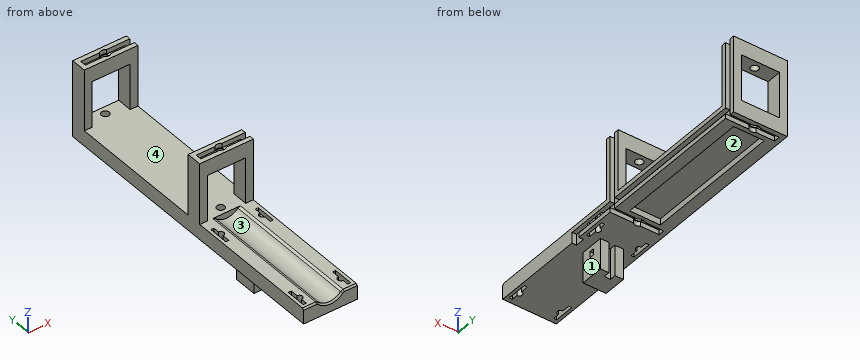
```python
from build123d import *

# Parameters (mm, degrees)
CYLINDER005_R     = 3
CYLINDER005_DEPTH = 3
CYLINDER006_R     = 3
CYLINDER006_DEPTH = 3
CYLINDER002_R     = 2.5
CYLINDER002_DEPTH = 60
BOX010_W          = 30
BOX010_H          = 4
BOX010_DEPTH      = 3
BOX008_W          = 30
BOX008_H          = 4
BOX008_DEPTH      = 3
BOX006_W          = 3
BOX006_H          = 4
BOX006_DEPTH      = 50
BOX004_W          = 3
BOX004_H          = 136
BOX004_DEPTH      = 4
BOX003_W          = 25
BOX003_H          = 220
BOX003_DEPTH      = 30
BOX002_W          = 35
BOX002_H          = 10
BOX002_DEPTH      = 50
BOX021_W          = 3
BOX021_H          = 6
BOX021_DEPTH      = 4
BOX018_W          = 20
BOX018_H          = 90
BOX018_DEPTH      = 4
CYLINDER008_R     = 2
CYLINDER008_DEPTH = 10
CYLINDER009_R     = 2
CYLINDER009_DEPTH = 10
CYLINDER010_R     = 2
CYLINDER010_DEPTH = 10
CYLINDER007_R     = 2
CYLINDER007_DEPTH = 10
BOX015_W          = 2
BOX015_H          = 13
BOX015_DEPTH      = 10
BOX016_W          = 2
BOX016_H          = 13
BOX016_DEPTH      = 10
BOX017_W          = 2
BOX017_H          = 13
BOX017_DEPTH      = 10
BOX014_W          = 2
BOX014_H          = 13
BOX014_DEPTH      = 10
CYLINDER003_R     = 3
CYLINDER003_DEPTH = 3
CYLINDER001_R     = 2.5
CYLINDER001_DEPTH = 60
BOX007_W          = 30
BOX007_H          = 4
BOX007_DEPTH      = 3
BOX005_W          = 3
BOX005_H          = 4
BOX005_DEPTH      = 50
CYLINDER_R        = 10
CYLINDER_DEPTH    = 90
BOX_W             = 35
BOX_H             = 200
BOX_DEPTH         = 10
CHAMFER_SIZE      = 1
BOX023_W          = 4
BOX023_H          = 4
BOX023_DEPTH      = 20
BOX022_W          = 20
BOX022_H          = 3
BOX022_DEPTH      = 4
BOX019_W          = 15
BOX019_H          = 15
BOX019_DEPTH      = 20
CYLINDER004_R     = 3
CYLINDER004_DEPTH = 3
BOX009_W          = 30
BOX009_H          = 4
BOX009_DEPTH      = 3
BOX001_W          = 35
BOX001_H          = 10
BOX001_DEPTH      = 50


with BuildPart() as cilindro005:
    # Cylinder005 → Cylinder005 (new body)
    with BuildSketch(Plane(origin=(17.5, 195, 0), x_dir=(1, 0, 0), z_dir=(0, 0, 1))):
        Circle(CYLINDER005_R)
    extrude(amount=CYLINDER005_DEPTH)


with BuildPart() as cilindro006:
    # Cylinder006 → Cylinder006 (new body)
    with BuildSketch(Plane(origin=(17.5, 195, 47), x_dir=(1, 0, 0), z_dir=(0, 0, 1))):
        Circle(CYLINDER006_R)
    extrude(amount=CYLINDER006_DEPTH)


with BuildPart() as cilindro002:
    # Cylinder002 → Cylinder002 (new body)
    with BuildSketch(Plane(origin=(17.5, 195, -1), x_dir=(1, 0, 0), z_dir=(0, 0, 1))):
        Circle(CYLINDER002_R)
    extrude(amount=CYLINDER002_DEPTH)


with BuildPart() as cubo010:
    # Box010 → Box010 (new body)
    with BuildSketch(Plane(origin=(3, 193, 47), x_dir=(1, 0, 0), z_dir=(0, 0, 1))):
        with Locations((15, 2)):
            Rectangle(BOX010_W, BOX010_H)
    extrude(amount=BOX010_DEPTH)


with BuildPart() as cubo008:
    # Box008 → Box008 (new body)
    with BuildSketch(Plane(origin=(3, 193, 0), x_dir=(1, 0, 0), z_dir=(0, 0, 1))):
        with Locations((15, 2)):
            Rectangle(BOX008_W, BOX008_H)
    extrude(amount=BOX008_DEPTH)


with BuildPart() as cubo006:
    # Box006 → Box006 (new body)
    with BuildSketch(Plane(origin=(32, 193, 0), x_dir=(1, 0, 0), z_dir=(0, 0, 1))):
        with Locations((1.5, 2)):
            Rectangle(BOX006_W, BOX006_H)
    extrude(amount=BOX006_DEPTH)


with BuildPart() as cubo004:
    # Box004 → Box004 (new body)
    with BuildSketch(Plane(origin=(32, 60, 3), x_dir=(1, 0, 0), z_dir=(0, 0, 1))):
        with Locations((1.5, 68)):
            Rectangle(BOX004_W, BOX004_H)
    extrude(amount=BOX004_DEPTH)


with BuildPart() as cubo003:
    # Box003 → Box003 (new body)
    with BuildSketch(Plane(origin=(5, 0, 10), x_dir=(1, 0, 0), z_dir=(0, 0, 1))):
        with Locations((12.5, 110)):
            Rectangle(BOX003_W, BOX003_H)
    extrude(amount=BOX003_DEPTH)


with BuildPart() as cut023:
    # Box002 → Box002 (new body)
    with BuildSketch(Plane(origin=(0, 190, 0), x_dir=(1, 0, 0), z_dir=(0, 0, 1))):
        with Locations((17.5, 5)):
            Rectangle(BOX002_W, BOX002_H)
    extrude(amount=BOX002_DEPTH)

    # Cut002: cut Cubo003
    add(cubo003.part, mode=Mode.SUBTRACT)

    # Cut005: cut Cubo004
    add(cubo004.part, mode=Mode.SUBTRACT)

    # Cut007: cut Cubo006
    add(cubo006.part, mode=Mode.SUBTRACT)

    # Cut011: cut Cubo008
    add(cubo008.part, mode=Mode.SUBTRACT)

    # Cut015: cut Cubo010
    add(cubo010.part, mode=Mode.SUBTRACT)

    # Cut017: cut Cilindro002
    add(cilindro002.part, mode=Mode.SUBTRACT)

    # Cut021: cut Cilindro006
    add(cilindro006.part, mode=Mode.SUBTRACT)

    # Cut023: cut Cilindro005
    add(cilindro005.part, mode=Mode.SUBTRACT)


with BuildPart() as cubo021:
    # Box021 → Box021 (new body)
    with BuildSketch(Plane(origin=(32, 60, 0), x_dir=(1, 0, 0), z_dir=(0, 0, 1))):
        with Locations((1.5, 3)):
            Rectangle(BOX021_W, BOX021_H)
    extrude(amount=BOX021_DEPTH)


with BuildPart() as cubo018:
    # Box018 → Box018 (new body)
    with BuildSketch(Plane(origin=(7.5, 100, 0), x_dir=(1, 0, 0), z_dir=(0, 0, 1))):
        with Locations((10, 45)):
            Rectangle(BOX018_W, BOX018_H)
    extrude(amount=BOX018_DEPTH)


with BuildPart() as cilindro008:
    # Cylinder008 → Cylinder008 (new body)
    with BuildSketch(Plane(origin=(31, 9, 0), x_dir=(1, 0, 0), z_dir=(0, 0, 1))):
        Circle(CYLINDER008_R)
    extrude(amount=CYLINDER008_DEPTH)


with BuildPart() as cilindro009:
    # Cylinder009 → Cylinder009 (new body)
    with BuildSketch(Plane(origin=(31, 77, 0), x_dir=(1, 0, 0), z_dir=(0, 0, 1))):
        Circle(CYLINDER009_R)
    extrude(amount=CYLINDER009_DEPTH)


with BuildPart() as cilindro010:
    # Cylinder010 → Cylinder010 (new body)
    with BuildSketch(Plane(origin=(4, 77, 0), x_dir=(1, 0, 0), z_dir=(0, 0, 1))):
        Circle(CYLINDER010_R)
    extrude(amount=CYLINDER010_DEPTH)


with BuildPart() as cilindro007:
    # Cylinder007 → Cylinder007 (new body)
    with BuildSketch(Plane(origin=(4, 9, 0), x_dir=(1, 0, 0), z_dir=(0, 0, 1))):
        Circle(CYLINDER007_R)
    extrude(amount=CYLINDER007_DEPTH)


with BuildPart() as cubo015:
    # Box015 → Box015 (new body)
    with BuildSketch(Plane(origin=(31, 3, 0), x_dir=(1, 0, 0), z_dir=(0, 0, 1))):
        with Locations((1, 6.5)):
            Rectangle(BOX015_W, BOX015_H)
    extrude(amount=BOX015_DEPTH)


with BuildPart() as cubo016:
    # Box016 → Box016 (new body)
    with BuildSketch(Plane(origin=(2, 70, 0), x_dir=(1, 0, 0), z_dir=(0, 0, 1))):
        with Locations((1, 6.5)):
            Rectangle(BOX016_W, BOX016_H)
    extrude(amount=BOX016_DEPTH)


with BuildPart() as cubo017:
    # Box017 → Box017 (new body)
    with BuildSketch(Plane(origin=(31, 70, 0), x_dir=(1, 0, 0), z_dir=(0, 0, 1))):
        with Locations((1, 6.5)):
            Rectangle(BOX017_W, BOX017_H)
    extrude(amount=BOX017_DEPTH)


with BuildPart() as cubo014:
    # Box014 → Box014 (new body)
    with BuildSketch(Plane(origin=(2, 3, 0), x_dir=(1, 0, 0), z_dir=(0, 0, 1))):
        with Locations((1, 6.5)):
            Rectangle(BOX014_W, BOX014_H)
    extrude(amount=BOX014_DEPTH)


with BuildPart() as cilindro003:
    # Cylinder003 → Cylinder003 (new body)
    with BuildSketch(Plane(origin=(17.5, 95, 0), x_dir=(1, 0, 0), z_dir=(0, 0, 1))):
        Circle(CYLINDER003_R)
    extrude(amount=CYLINDER003_DEPTH)


with BuildPart() as cilindro001:
    # Cylinder001 → Cylinder001 (new body)
    with BuildSketch(Plane(origin=(17.5, 95, -1), x_dir=(1, 0, 0), z_dir=(0, 0, 1))):
        Circle(CYLINDER001_R)
    extrude(amount=CYLINDER001_DEPTH)


with BuildPart() as cubo007:
    # Box007 → Box007 (new body)
    with BuildSketch(Plane(origin=(3, 93, 0), x_dir=(1, 0, 0), z_dir=(0, 0, 1))):
        with Locations((15, 2)):
            Rectangle(BOX007_W, BOX007_H)
    extrude(amount=BOX007_DEPTH)


with BuildPart() as cubo005:
    # Box005 → Box005 (new body)
    with BuildSketch(Plane(origin=(32, 93, 0), x_dir=(1, 0, 0), z_dir=(0, 0, 1))):
        with Locations((1.5, 2)):
            Rectangle(BOX005_W, BOX005_H)
    extrude(amount=BOX005_DEPTH)


with BuildPart() as cilindro:
    # Cylinder → Cylinder (new body)
    with BuildSketch(Plane(origin=(17.5, 0, 16), x_dir=(1, 0, 0), z_dir=(0, 1, 0))):
        Circle(CYLINDER_R)
    extrude(amount=CYLINDER_DEPTH)


with BuildPart() as cut037:
    # Box → Box (new body)
    with BuildSketch(Plane.XY):
        with Locations((17.5, 100)):
            Rectangle(BOX_W, BOX_H)
    extrude(amount=BOX_DEPTH)

    # Cut: cut Cilindro
    add(cilindro.part, mode=Mode.SUBTRACT)

    # Chamfer
    chamfer_edges = [cut037.edges().sort_by_distance(p)[0] for p in [
        (30.25, 0, 10),
        (17.5, 0, 6),
        (4.75, 0, 10),
        (25.5, 45, 10),
        (9.5, 45, 10),
    ]]
    chamfer(chamfer_edges, length=CHAMFER_SIZE)

    # Cut003: cut Cubo004
    add(cubo004.part, mode=Mode.SUBTRACT)

    # Cut008: cut Cubo005
    add(cubo005.part, mode=Mode.SUBTRACT)

    # Cut009: cut Cubo006
    add(cubo006.part, mode=Mode.SUBTRACT)

    # Cut012: cut Cubo007
    add(cubo007.part, mode=Mode.SUBTRACT)

    # Cut013: cut Cubo008
    add(cubo008.part, mode=Mode.SUBTRACT)

    # Cut018: cut Cilindro001
    add(cilindro001.part, mode=Mode.SUBTRACT)

    # Cut019: cut Cilindro002
    add(cilindro002.part, mode=Mode.SUBTRACT)

    # Cut024: cut Cilindro003
    add(cilindro003.part, mode=Mode.SUBTRACT)

    # Cut025: cut Cilindro005
    add(cilindro005.part, mode=Mode.SUBTRACT)

    # Cut028: cut Cubo014
    add(cubo014.part, mode=Mode.SUBTRACT)

    # Cut029: cut Cubo017
    add(cubo017.part, mode=Mode.SUBTRACT)

    # Cut030: cut Cubo016
    add(cubo016.part, mode=Mode.SUBTRACT)

    # Cut031: cut Cubo015
    add(cubo015.part, mode=Mode.SUBTRACT)

    # Cut032: cut Cilindro007
    add(cilindro007.part, mode=Mode.SUBTRACT)

    # Cut033: cut Cilindro010
    add(cilindro010.part, mode=Mode.SUBTRACT)

    # Cut034: cut Cilindro009
    add(cilindro009.part, mode=Mode.SUBTRACT)

    # Cut035: cut Cilindro008
    add(cilindro008.part, mode=Mode.SUBTRACT)

    # Cut036: cut Cubo018
    add(cubo018.part, mode=Mode.SUBTRACT)

    # Cut037: cut Cubo021
    add(cubo021.part, mode=Mode.SUBTRACT)


with BuildPart() as cubo023:
    # Box023 → Box023 (new body)
    with BuildSketch(Plane(origin=(16, 61, -20), x_dir=(1, 0, 0), z_dir=(0, 0, 1))):
        with Locations((2, 2)):
            Rectangle(BOX023_W, BOX023_H)
    extrude(amount=BOX023_DEPTH)


with BuildPart() as cubo022:
    # Box022 → Box022 (new body)
    with BuildSketch(Plane(origin=(8, 56, -7), x_dir=(1, 0, 0), z_dir=(0, 0, 1))):
        with Locations((10, 1.5)):
            Rectangle(BOX022_W, BOX022_H)
    extrude(amount=BOX022_DEPTH)


with BuildPart() as cut039:
    # Box019 → Box019 (new body)
    with BuildSketch(Plane(origin=(10.5, 50, -20), x_dir=(1, 0, 0), z_dir=(0, 0, 1))):
        with Locations((7.5, 7.5)):
            Rectangle(BOX019_W, BOX019_H)
    extrude(amount=BOX019_DEPTH)

    # Cut038: cut Cubo022
    add(cubo022.part, mode=Mode.SUBTRACT)

    # Cut039: cut Cubo023
    add(cubo023.part, mode=Mode.SUBTRACT)


with BuildPart() as cut039_1:
    # Cut039 placement: moved
    add(cut039.part.moved(Location((0, 7, 0))))


with BuildPart() as cilindro004:
    # Cylinder004 → Cylinder004 (new body)
    with BuildSketch(Plane(origin=(17.5, 95, 47), x_dir=(1, 0, 0), z_dir=(0, 0, 1))):
        Circle(CYLINDER004_R)
    extrude(amount=CYLINDER004_DEPTH)


with BuildPart() as cubo009:
    # Box009 → Box009 (new body)
    with BuildSketch(Plane(origin=(3, 93, 47), x_dir=(1, 0, 0), z_dir=(0, 0, 1))):
        with Locations((15, 2)):
            Rectangle(BOX009_W, BOX009_H)
    extrude(amount=BOX009_DEPTH)


with BuildPart() as fusion:
    # Box001 → Box001 (new body)
    with BuildSketch(Plane(origin=(0, 90, 0), x_dir=(1, 0, 0), z_dir=(0, 0, 1))):
        with Locations((17.5, 5)):
            Rectangle(BOX001_W, BOX001_H)
    extrude(amount=BOX001_DEPTH)

    # Cut001: cut Cubo003
    add(cubo003.part, mode=Mode.SUBTRACT)

    # Cut004: cut Cubo004
    add(cubo004.part, mode=Mode.SUBTRACT)

    # Cut006: cut Cubo005
    add(cubo005.part, mode=Mode.SUBTRACT)

    # Cut010: cut Cubo007
    add(cubo007.part, mode=Mode.SUBTRACT)

    # Cut014: cut Cubo009
    add(cubo009.part, mode=Mode.SUBTRACT)

    # Cut016: cut Cilindro001
    add(cilindro001.part, mode=Mode.SUBTRACT)

    # Cut020: cut Cilindro004
    add(cilindro004.part, mode=Mode.SUBTRACT)

    # Cut022: cut Cilindro003
    add(cilindro003.part, mode=Mode.SUBTRACT)

    # Fusion: union Cut023, Cut037, Cut039
    add(cut023.part)
    add(cut037.part)
    add(cut039_1.part)


solid = fusion.part
```
The listing builds one solid part. Answer for the finished solid, in the listing's coordinates (mm). Face numbers are marked on the shaded views. A direction names the side the tool comes from. Give positions to 0.01 mm unless a question says otherwise; leave off trailing zeros. Order: outer loops, then holes, each group sorted by start corner. A loop starts at its lowest first (then second) coordinate and runs counter-clockwise, first axis right, second up. Notation, with made-up numbers: (29, 49.5) -> (33, 49.5) arc R11 cw to (33, 69.5) -> close; hole circle Ø1 at (63, 70). An arc over 180 degrees is marked (long way). Write each question's results on one line, items separated by ' | '.
Q1. The part is cut by section B-B, the plane z = 17.5. Give the vertices of the cut face in (x, y).
Checked values:
outline: (0, 90) -> (5, 90) -> (5, 100) -> (0, 100) -> close; (0, 190) -> (5, 190) -> (5, 200) -> (0, 200) -> close; (30, 90) -> (35, 90) -> (35, 93) -> (32, 93) -> (32, 97) -> (35, 97) -> (35, 100) -> (30, 100) -> close; (30, 190) -> (35, 190) -> (35, 193) -> (32, 193) -> (32, 197) -> (35, 197) -> (35, 200) -> (30, 200) -> close
Q2. Determine the mould class of the marked faces 1 and 2 for opening direction X: pulls with the +X half, pulls with the -X half, needs draft (parallel to the pull), parting line crosses it, or undercut.
Checked values:
face 1: pulls with the +X half | face 2: undercut
Q3. The part is cut by section C-C, the plane y = 195. Give the vertices of the cut face in (x, z), and give its area (3 significant figures).
Checked values:
outline: (0, 0) -> (3, 0) -> (3, 3) -> (15, 3) -> (15, 10) -> (5, 10) -> (5, 40) -> (15, 40) -> (15, 47) -> (3, 47) -> (3, 50) -> (0, 50) -> close; (20, 3) -> (32, 3) -> (32, 47) -> (20, 47) -> (20, 40) -> (30, 40) -> (30, 10) -> (20, 10) -> close | area: 606 mm^2
Q4. The part is cut by section D-D, the plane x = 12.5. State how many separate pieces and enclosed holes the cut face has, and give its area (3 significant figures).
Checked values:
separate pieces: 3 | enclosed holes: 1 | area: 1,840 mm^2
Q5. The part is cut by section A-A, the plane y = 77. Give the vertices of the cut face in (x, z).
Checked values:
outline: (0, 0) -> (2, 0) -> (2, 10) -> (0, 10) -> close; (6, 0) -> (29, 0) -> (29, 10) -> (26.5, 10) -> (24.86, 9.23) arc R10 cw to (10.14, 9.23) -> (8.5, 10) -> (6, 10) -> close; (33, 0) -> (35, 0) -> (35, 3) -> (33, 3) -> close; (33, 7) -> (35, 7) -> (35, 10) -> (33, 10) -> close
Q6. Straight lines are drawn through the part: probe 1 along Y at (x, z) = (17.5, 42); probe 2 along X at (y, z) = (95, 5); probe 3 along Y at (x, z) = (17.5, 4.5). For each, find the intervals that lie inside material, in ascending order. Write a range as from..to.
Checked values:
probe 1: y = 90..92.5, 97.5..100, 190..192.5, 197.5..200 | probe 2: x = 0..15, 20..32 | probe 3: y = 0..92.5, 97.5..192.5, 197.5..200
Q7. Which of the six approach directions +Z, -Z, +X, -X, +Y, -Y give full straight-line access (tool end or side, diameter ignored) to the marked faces 3 and 4?
Checked values:
face 3: +Z, -Y | face 4: none
Q8. Each of these flat-tipped pins is pushed along its axis until it touches: P1, Ø1.5, axis at y = 73, z = 3.5, coming from the -X side; P2, Ø6, axis at x = 23.5, z = -10.5, coming from the +Y side; P3, Ø10, axis at x = 20, y = 135, coming from the -Z side; P4, Ø12, axis at x = 29, y = 27, coming from the +Z side. Where does it stop, or does it pass through?
Checked values:
P1: stops at x = 0 | P2: stops at y = 72 | P3: stops at z = 4 | P4: stops at z = 10
